Verification items for this drawing (mm, ordinates from the low corner). A direction names the side the tool comes from. Round coordinates to 2 decimals unless told otherwise and drop trailing zeros. Loops run counter-clockwise (first coordinate to the right, second up) from the corner with the lowest first, then second, coordinate; pieces in that order, holes last. Notation, with made-up numbers: M 5.25,2.5 L 59.25,2.5 A15 cw 59.25,12.5 Z; hole C 15,-3.75 d3. An arc over 180 degrees is marked long. Answer as CSV lines item,"result".
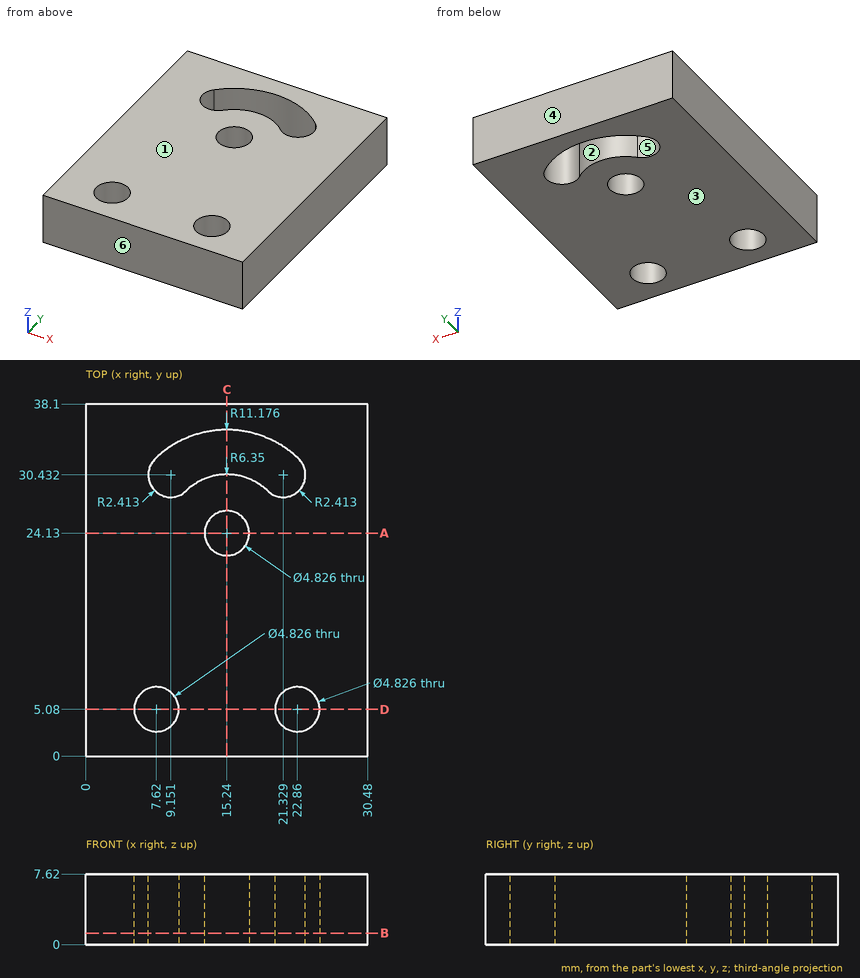
1) Draft check along Y on the marked faces 3, 4, 5 and 6. Enter one of: +Y half, -Y half, draft (parallel to the pull), parting line (faces both ways), or undercut.
Here are the results:
face 3,"draft"
face 4,"+Y half"
face 5,"undercut"
face 6,"-Y half"
2) Section check C-C (x = 15.24). Record the cut outline in (y, z).
Here are the results:
outline,"M 0,0 L 21.72,0 L 21.72,7.62 L 0,7.62 Z; M 26.54,0 L 30.48,0 L 30.48,7.62 L 26.54,7.62 Z; M 35.31,0 L 38.1,0 L 38.1,7.62 L 35.31,7.62 Z"
3) Section check A-A (y = 24.13). Record the cut outline in (x, z).
Here are the results:
outline,"M 0,0 L 12.83,0 L 12.83,7.62 L 0,7.62 Z; M 17.65,0 L 30.48,0 L 30.48,7.62 L 17.65,7.62 Z"
4) Material ranges on probe 1 along Y at (x, z) = (17, 1.25); probe 2 along Y at (x, z) = (7.62, 2) (1 decimal); probe 3 along Y at (x, z) = (6.5, 3), recorded low to high.
Here are the results:
probe 1,"y = 0 to 22.48, 25.78 to 30.23, 35.17 to 38.1"
probe 2,"y = 0 to 2.7, 7.5 to 28.6, 32.3 to 38.1"
probe 3,"y = 0 to 2.94, 7.22 to 38.1"
5) Section check B-B (z = 1.25). Record the cut outline in (x, y), plus the area to 3 significant figures.
Here are the results:
outline,"M 0,0 L 30.48,0 L 30.48,38.1 L 0,38.1 Z; hole C 7.62,5.08 d4.83; hole M 7.47,32.17 A2.41 ccw 10.83,28.7 A6.35 cw 19.65,28.7 A2.41 ccw 23.01,32.17 A11.18 ccw Z; hole C 15.24,24.13 d4.83; hole C 22.86,5.08 d4.83"
area,"1,020 mm^2"
6) Set-up check for the marked faces 1 and 2: record each of +Z, -Z, +X, -X, +Y, -Y from which the full face is reachable in a straight line by a thin tool's end or side.
Here are the results:
face 1,"+Z, +X, -X, +Y, -Y"
face 2,"+Z, -Z"
7) Section check D-D (y = 5.08). Record the cut outline in (x, z).
Here are the results:
outline,"M 0,0 L 5.21,0 L 5.21,7.62 L 0,7.62 Z; M 10.03,0 L 20.45,0 L 20.45,7.62 L 10.03,7.62 Z; M 25.27,0 L 30.48,0 L 30.48,7.62 L 25.27,7.62 Z"
8) Go/stop test with a flat-tipped pin: pin 1 (4 mm diameter, centred on x = 15.24, y = 24.13, fed in from -Z). Record where the tip stops, or that it passes through.
Here are the results:
pin 1,"passes through"
